Read the model definition and answer for the solid it produces. Units are mm, in the model's axes. Coordinates: 2 decimals unless noted, no trailing zeros. Loops run counter-clockwise (first coordinate to the right, second up) from the corner with the lowest first, then second, coordinate; pieces in that order, holes last.
from build123d import *

# Parameters (mm, degrees)
F1_DEPTH = 101.6
F2_R     = 11.6260505805
F3_DEPTH = 88.9
F5_DEPTH = 25.4


with BuildPart() as f1:
    # F0 (on Front) → F1 (new body)
    with BuildSketch(Plane.XZ):
        Polygon((39.3597595394, 28.3906441182), (-35.6722733648, 28.3906441182), (-35.6722733648, -50.6975799799), (39.3597595394, -50.6975799799), (79.9182447382, -50.6975799799), align=None)
    extrude(amount=F1_DEPTH)

    # F2 (on Right) → F3 (cut, symmetric)
    with BuildSketch(Plane.YZ):
        with Locations((-51.2301623821, -11.2456455827)):
            Circle(F2_R)
    extrude(amount=F3_DEPTH, both=True, mode=Mode.SUBTRACT)

    # F4 (on Front) → F5 (join)
    with BuildSketch(Plane.XZ):
        Polygon((-35.5649143457, 35.2117754519), (-35.5649143457, -50.3288730979), (87.5841230154, -50.3288730979), (42.7858941257, 35.2117754519), align=None)
    extrude(amount=F5_DEPTH)


solid = f1.part
Item 1: A cutting plane is placed at B-B on x = 0.5. Determine the outline of the cut face in (y, z).
Numbers:
outline: (-101.6, -50.7) - (0, -50.7) - (0, 35.21) - (-25.4, 35.21) - (-25.4, 28.39) - (-101.6, 28.39) - close; hole circle Ø23.25 at (-51.23, -11.25)
Item 2: Find the intervals of material crossed by line 1 along Y through (x, z) = (20.5, -11.5); line 2 along Z through (x, y) = (-10, -94); line 3 along Y through (x, z) = (6.5, -10), in increasing order.
Numbers:
line 1: y = -101.6 to -62.85, -39.61 to 0
line 2: z = -50.7 to 28.39
line 3: y = -101.6 to -62.79, -39.67 to 0
Item 3: Determine the mould class of faces 1 (the face through (15.697, -45.865, -21.56)), 2 (the face through (49, -25.4, 12)), 3 (the face through (65.5, -12.52, -8.16)) for opening direction Z: released by +Z, released by -Z, zero draft, split by the parting line, or undercut.
Numbers:
face 1: undercut
face 2: zero draft
face 3: released by +Z
Item 4: Given pin 1 (2.5 mm diameter, centred on x = 83, y = -13, fed in from -Z); pin 2 (10 mm diameter, centred on y = -67.5, z = -5.5, fed in from +X); pin 3 (3 mm diameter, centred on x = -6, y = -83.5, fed in from +Z), each flat-ended and moving along its own axis, determine where each tip first touches the part or whether it passes through.
Numbers:
pin 1: stops at z = -50.33
pin 2: stops at x = 59.3
pin 3: stops at z = 28.39
Item 5: A cutting plane is placed at A-A on y = -55. Determine the outline of the cut face in (x, z), then the cut area to 3 significant figures.
Numbers:
outline: (-35.67, -50.7) - (79.92, -50.7) - (65.33, -22.24) - (-35.67, -22.24) - close; (-35.67, -0.25) - (54.05, -0.25) - (39.36, 28.39) - (-35.67, 28.39) - close
area: 5,440 mm2
Item 6: A cutting plane is placed at D-D on z = 16. Determine the outline of the cut face in (x, y).
Numbers:
outline: (-35.67, -101.6) - (45.71, -101.6) - (45.71, -25.4) - (52.85, -25.4) - (52.85, 0) - (-35.67, 0) - close
Item 7: A cutting plane is placed at C-C on y = -11. Determine the outline of the cut face in (x, z).
Numbers:
outline: (-35.67, -50.7) - (79.92, -50.7) - (79.73, -50.33) - (87.58, -50.33) - (42.79, 35.21) - (-35.56, 35.21) - (-35.56, 28.39) - (-35.67, 28.39) - close
